The model under review builds one solid part; all positions refer to its coordinate system, in mm. Face numbers are marked on the shaded views. A direction names the side the tool comes from. Round coordinates to 2 decimals unless told otherwise and drop trailing zeros. Order: outer loops, then holes, each group sorted by start corner. A loop starts at its lowest first (then second) coordinate and runs counter-clockwise, first axis right, second up. Notation, with made-up numbers: M 2.5,79.5 L 20.5,79.5 A22 ccw 20.5,87.5 Z; hole C 11,-34 d2. An arc over 180 degrees is marked long. Answer as a JSON object with one key per item and string values. Group by question number.
1. Add section B-B on x = 0. State the section outline as (y, z) points (3 decimals).
2. Add section D-D on x = 19.5. State the section outline as (y, z) points.
3. Clearance check with flat-ended pins moving along their axes: P1, Ø3, axis at y = 0, z = 7, coming from the +X side (3 decimals); P2, Ø3, axis at x = 13, y = 2, coming from the -Z side; P3, Ø1.5, axis at x = -19.5, z = 6, coming from the +Y side (3 decimals). State where each tip first meets the part, or that it passes through.
4. Add section C-C on y = 0. State the section outline as (x, z) points (3 decimals), and give its area (3 significant figures).
5. Machinability: for the marked faces 1 and 2, which of the approach directions +Z, -Z, +X, -X, +Y, -Y give a long, thin tool a straight path to every point of the face, cutting with its end or side? Answer none if there is none.
6. Add section A-A on z = 9.75. State the section outline as (x, y) points (3 decimals).
7. To check wall thickness, follow probe 1 along X at (y, z) = (1.25, 11.25); probe 2 along X at (y, z) = (-1.5, 4.25); probe 3 along Z at (x, y) = (-6, 3.25). State the ranges of each line that lie inside material, in increasing order. Write a range as [from, to].
8. Mouldability with a two-part tool opening along X and no side actions: class the marked faces 3, 4 and 5 as released by +X, released by -X, zero draft, split by the parting line, or undercut.
```python
from build123d import *

# Parameters (mm, degrees)
SKETCH1_R             = 3.175
BOSS_EXTRUDE1_DEPTH   = 12.7
BOSS_EXTRUDE1_2_DEPTH = 12.7
BOSS_EXTRUDE1_3_DEPTH = 12.7
SKETCH2_W             = 50.8
SKETCH2_H             = 12.7
BOSS_EXTRUDE2_DEPTH   = 6.35


with BuildPart() as part:
    # Sketch1 → Boss-Extrude1 (new body)
    with BuildSketch(Plane.XY):
        Circle(SKETCH1_R)
    extrude(amount=BOSS_EXTRUDE1_DEPTH)



with BuildPart() as body_2:
    # Sketch1 → Boss-Extrude1 2 (new body)
    with BuildSketch(Plane.XY):
        with Locations((19.05, 0)):
            Circle(SKETCH1_R)
    extrude(amount=BOSS_EXTRUDE1_2_DEPTH)


with BuildPart() as body_3:
    # Sketch1 → Boss-Extrude1 3 (new body)
    with BuildSketch(Plane.XY):
        with Locations((-19.05, 0)):
            Circle(SKETCH1_R)
    extrude(amount=BOSS_EXTRUDE1_3_DEPTH)


with BuildPart() as part_1:
    add(part.part)

    add(body_2.part)  # Boss-Extrude2 merges body 2

    add(body_3.part)  # Boss-Extrude2 merges body 3
    # Sketch2 → Boss-Extrude2 (add)
    with BuildSketch(Plane.XY.offset(12.7)):
        Rectangle(SKETCH2_W, SKETCH2_H)
    extrude(amount=BOSS_EXTRUDE2_DEPTH)


solid = part_1.part
```
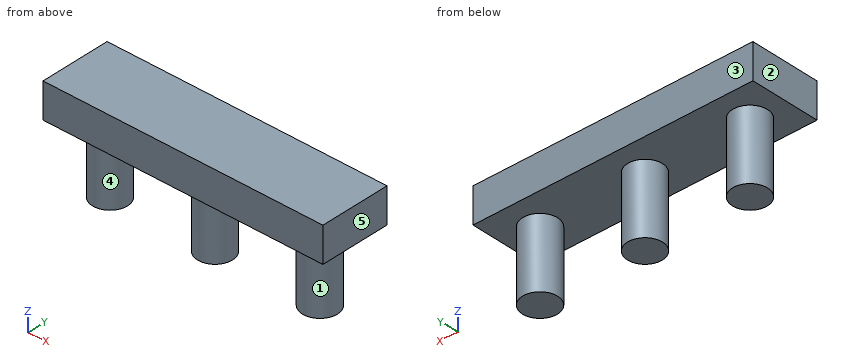
Recorded:
{
 "1": {"outline": "M -6.35,12.7 L -3.175,12.7 L -3.175,0 L 3.175,0 L 3.175,12.7 L 6.35,12.7 L 6.35,19.05 L -6.35,19.05 Z"},
 "2": {"outline": "M -6.35,12.7 L -3.14,12.7 L -3.14,0 L 3.14,0 L 3.14,12.7 L 6.35,12.7 L 6.35,19.05 L -6.35,19.05 Z"},
 "3": {"P1": "stops at x = 22.225", "P2": "stops at z = 12.7", "P3": "stops at y = 3.175"},
 "4": {"outline": "M -25.4,12.7 L -22.225,12.7 L -22.225,0 L -15.875,0 L -15.875,12.7 L -3.175,12.7 L -3.175,0 L 3.175,0 L 3.175,12.7 L 15.875,12.7 L 15.875,0 L 22.225,0 L 22.225,12.7 L 25.4,12.7 L 25.4,19.05 L -25.4,19.05 Z", "area": "565 mm²"},
 "5": {"face 1": "-Z", "face 2": "+Z, -Z, -X, +Y, -Y"},
 "6": {"outline": "C -19.05,0 d6.35; C 0,0 d6.35; C 19.05,0 d6.35"},
 "7": {"probe 1": "x = [-21.97, -16.13], [-2.92, 2.92], [16.13, 21.97]", "probe 2": "x = [-21.85, -16.25], [-2.8, 2.8], [16.25, 21.85]", "probe 3": "z = [12.7, 19.05]"},
 "8": {"face 3": "zero draft", "face 4": "undercut", "face 5": "released by +X"}
}
